Source: CAD feature listing. Evaluate the final solid. Frame: model axes, mm. Round coordinates to 2 decimals unless told otherwise and drop trailing zeros. Write each loop counter-clockwise with the first axis right and the second up, starting at its lowest first coordinate (ties: lowest second). Pieces come first, ordered by that corner, then holes. Notation, with made-up numbers: M 53.25,78 L 97.25,78 A14 ccw 97.25,102 Z; hole C -34.75,81 d10. An arc over 180 degrees is marked long. Answer in a Markdown table with one row per item. Add a question column.
Item 1: Contact query for flat-ended pins moving along their axis: pin 1 (1.5 mm diameter, centred on x = 0.5, z = 408.5, fed in from +Y); pin 2 (2.5 mm diameter, centred on x = 3.5, z = 168.5, fed in from -Y); pin 3 (6 mm diameter, centred on y = 13.5, z = 308, fed in from +X) (3 decimals). Output: stop coordinate, or through.
Item 2: Material intervals for probe 1 along X at (y, z) = (4.5, 284.5) (3 decimals); probe 2 along Y at (x, z) = (2.5, 236.5); probe 3 along X at (y, z) = (19.75, 49.5), sorted ascending.
Item 3: Cut plane A-A on z = 457.5. Return loops of the section in (x, y) (3 decimals), and give its area (3 significant figures).
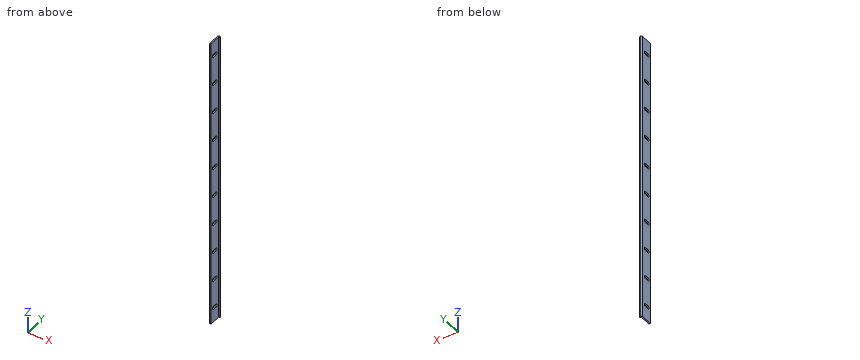
from build123d import *

# Parameters (mm, degrees)
BOSS_EXTRUDE1_DEPTH = 500
CUT_EXTRUDE1_DEPTH  = 3.375
LPATTERN1_COUNT     = 10
LPATTERN1_PITCH     = 50


with BuildPart() as part:
    # Sketch1 → Boss-Extrude1 (new body)
    with BuildSketch(Plane.XY):
        with BuildLine():
            Line((0, 0.3), (0, 20.125))
            ThreePointArc((0, 20.125), (0.02283614, 20.23980503), (0.087867966, 20.337132034))
            Line((0.087867966, 20.337132034), (2.162867966, 22.412132034))
            ThreePointArc((2.162867966, 22.412132034), (2.375, 22.5), (2.587132034, 22.412132034))
            Line((2.587132034, 22.412132034), (4.662132034, 20.337132034))
            ThreePointArc((4.662132034, 20.337132034), (4.72716386, 20.23980503), (4.75, 20.125))
            Line((4.75, 20.125), (4.75, 19.85))
            ThreePointArc((4.75, 19.85), (4.662132034, 19.637867966), (4.45, 19.55))
            Line((4.45, 19.55), (2.375, 19.55))
            Line((2.375, 19.55), (2.375, 0.3))
            ThreePointArc((2.375, 0.3), (2.287132034, 0.087867966), (2.075, 0))
            Line((2.075, 0), (0.3, 0))
            ThreePointArc((0.3, 0), (0.087867966, 0.087867966), (0, 0.3))
        make_face()
    extrude(amount=BOSS_EXTRUDE1_DEPTH)

    # Sketch2 → Cut-Extrude1 (cut, through all)
    with BuildSketch(Plane(origin=(2.375, 0, 0), x_dir=(0, 0, -1), z_dir=(1, 0, 0))):
        with BuildLine():
            Line((-22.35, 12.7), (-22.35, 6))
            ThreePointArc((-22.35, 6), (-25, 3.35), (-27.65, 6))
            Line((-27.65, 6), (-27.65, 12.7))
            ThreePointArc((-27.65, 12.7), (-25, 15.35), (-22.35, 12.7))
        make_face()
    cut_extrude1 = extrude(amount=-CUT_EXTRUDE1_DEPTH, mode=Mode.SUBTRACT)

    # LPattern1: Cut-Extrude1 ×10
    with Locations(*[(0, 0, i * LPATTERN1_PITCH) for i in range(1, LPATTERN1_COUNT)]):
        add(cut_extrude1, mode=Mode.SUBTRACT)


solid = part.part
Results below:
| question | item | result |
|---|---|---|
| 1 | pin 1 | y = 21.5 |
| 1 | pin 2 | y = 0.06 |
| 1 | pin 3 | x = 2.375 |
| 2 | probe 1 | 0 to 2.375 |
| 2 | probe 2 | 19.55 to 22.47 |
| 2 | probe 3 | 0 to 4.73 |
| 3 | outline | M 0,0.3 A0.3 ccw 0.3,0 L 2.075,0 A0.3 ccw 2.375,0.3 L 2.375,19.55 L 4.45,19.55 A0.3 ccw 4.75,19.85 L 4.75,20.125 A0.3 ccw 4.662,20.337 L 2.587,22.412 A0.3 ccw 2.163,22.412 L 0.088,20.337 A0.3 ccw 0,20.125 Z |
| 3 | area | 55.3 mm2 |
